Read the model definition and answer for the solid it produces. Units are mm, in the model's axes. Round coordinates to 2 decimals unless told otherwise and drop trailing zeros. Loops run counter-clockwise (first coordinate to the right, second up) from the corner with the lowest first, then second, coordinate; pieces in that order, holes last. Notation, with made-up numbers: (18.5, 78.5) - (28.5, 78.5) arc R13 cw to (28.5, 85.5) - close; hole circle Ø10 at (81.5, -15.75). An arc over 180 degrees is marked (long way). Use CSV: the item, a comma, the result in double quotes. Start each with the question number.
1. Find section C-C (z = 0.9). Give the vertices of the cut face in (x, y), and give its area (3 significant figures).
2. Find section B-B (x = 22.5). Give the vertices of the cut face in (y, z), and give its area (3 significant figures).
3. Determine the mould class of faces 1 (the flat face through (0, 3, 1)), 2 (the cylindrical face through (21.013, 2.695, 0.986)), 3 (the cylindrical face through (1.235, 1.694, 0.986)), 4 (the flat face through (13, 5, 1)) for opening direction X: +X half, -X half, draft (parallel to the pull), parting line (faces both ways), or undercut.
4. Find section D-D (y = 1.35). Give the vertices of the cut face in (x, z).
5. Consider line 1 along X through (y, z) = (2.5, 1.05); line 2 along X through (y, z) = (1.35, 1.1); line 3 along Y through (x, z) = (22.5, 1.55). Determine where each line is inside the solid, lowest interval first.
6. Given pin 1 Ø2 at (x, y) = (13, 3.5) entering from -Z, flat-ended and moving along its own axis, determine where the tip first touches the part or whether it passes through.
7. Find section A-A (y = 2.5). Give the vertices of the cut face in (x, z), and give its area (3 significant figures).
Autodesk Inventor part; units mm, degrees
ref_plane "YZ Plane" through (0, 0, 0) normal (1, 0, 0) x (0, 1, 0)
ref_plane "XZ Plane" through (0, 0, 0) normal (0, 1, 0) x (-1, 0, 0)
ref_plane "XY Plane" through (0, 0, 0) normal (0, 0, 1) x (1, 0, 0)
sketch "スケッチ1" plane through (0, 0, 0) normal (0, 0, 1) x (1, 0, 0)
  line L0 (0, 0) -> (25, 0)
  line L1 (25, 0) -> (25, 5)
  line L2 (25, 5) -> (0, 5)
  line L3 (0, 5) -> (0, 0)
  dimension "d0" = 25
  dimension "d1" = 5
extrude "押し出し1" add sketch "スケッチ1" along normal blind 2
sketch "スケッチ2" plane through (0, 0, 2) normal (0, 0, 1) x (1, 0, 0)
  line L0 (0, 5) -> (0, 0)
  line L1 (25, 0) -> (25, 5)
  point P0 (2.5, 2.5)
  point P1 (22.5, 2.5)
  dimension "d4" = 2.5
  dimension "d5" = 2.5
hole "穴1" at (2.5, 2.5, 2) at (22.5, 2.5, 2) direction (0, 0, -1) diameter 3 end through all
properties part number "短いの"
Filled sheet:
1,outline,"(0, 0) - (25, 0) - (25, 5) - (0, 5) - close; hole circle Ø3 at (2.5, 2.5); hole circle Ø3 at (22.5, 2.5)"
1,area,"111 mm²"
2,outline,"(0, 0) - (1, 0) - (1, 2) - (0, 2) - close; (4, 0) - (5, 0) - (5, 2) - (4, 2) - close"
2,area,"4.00 mm²"
3,face 1,"-X half"
3,face 2,"undercut"
3,face 3,"undercut"
3,face 4,"draft"
4,outline,"(0, 0) - (1.54, 0) - (1.54, 2) - (0, 2) - close; (3.46, 0) - (21.54, 0) - (21.54, 2) - (3.46, 2) - close; (23.46, 0) - (25, 0) - (25, 2) - (23.46, 2) - close"
5,line 1,"x = 0 to 1, 4 to 21, 24 to 25"
5,line 2,"x = 0 to 1.54, 3.46 to 21.54, 23.46 to 25"
5,line 3,"y = 0 to 1, 4 to 5"
6,pin 1,"stops at z = 0"
7,outline,"(0, 0) - (1, 0) - (1, 2) - (0, 2) - close; (4, 0) - (21, 0) - (21, 2) - (4, 2) - close; (24, 0) - (25, 0) - (25, 2) - (24, 2) - close"
7,area,"38.0 mm²"
